Check sheet for the modelled part. Datum: model origin and axes. Units: mm. Round coordinates to 2 decimals unless told otherwise and drop trailing zeros.
Item 1: Material ranges on line 1 (Y direction, x = 0, z = 137); line 2 (X direction, y = -4.5, z = 201), recorded low to high.
Item 2: Release check for a two-part mould opening along X. For faces 1 (the cylindrical face through (-0.596, 2.685, 108.46)), 2 (the flat face through (6, 10, 108)), 3 (the flat face through (10, -6, 108)) record: +X half, -X half, draft (parallel to the pull), parting line (faces both ways), or undercut.
Item 3: Go/stop test with flat-tipped pins: pin 1 Ø3 at (x, y) = (2, -6) entering from +Z; pin 2 Ø1.5 at (y, z) = (0, 160.5) entering from +X; pin 3 Ø0.8 at (y, z) = (2, 73.5) entering from -X. Record where each tip stops, or that it passes through.
Autodesk Inventor part; units mm, degrees
ref_plane "Startebene" through (0, 0, 0) normal (0, 0, 1) x (1, 0, 0)
ref_plane "Endebene" through (0, 0, 320) normal (0, 0, 1) x (1, 0, 0)
ref_plane "Startebene1" through (0, 0, 0) normal (0, 0, 1) x (1, 0, 0)
ref_plane "Startebene" through (0, 0, 0) normal (0, 0, 1) x (1, 0, 0)
ref_plane "Endebene" through (0, 0, 320) normal (0, 0, 1) x (1, 0, 0)
ref_plane "Startebene1" through (0, 0, 0) normal (0, 0, 1) x (1, 0, 0)
ref_plane "Endebene1" through (0, 0, 220) normal (0, 0, 1) x (1, 0, 0)
ref_plane "Startebene2" through (0, 0, 0) normal (0, 0, 1) x (1, 0, 0)
ref_plane "Endebene2" through (0, 0, 220) normal (0, 0, 1) x (1, 0, 0)
sketch "Skizze" plane through (0, 0, 0) normal (0, 0, 1) x (1, 0, 0)
  line L0 (-10, 9) -> (-10, 3.3)
  arc A0 (-10, 3.3) -> (-9.7, 3) centre (-9.7, 3.3) ccw
  line L1 (-9.7, 3) -> (-8, 3)
  line L2 (-8, 3) -> (-8, 6)
  line L3 (-8, 6) -> (-7.0607, 6)
  line L4 (-7.0607, 6) -> (-4, 2.9393)
  line L5 (-4, 2.9393) -> (-4, 0.3)
  line L6 (-4, 0.3) -> (-3.7, 0)
  line L7 (-3.7, 0) -> (-4, -0.3)
  line L8 (-4, -0.3) -> (-4, -2.9393)
  line L9 (-4, -2.9393) -> (-7.0607, -6)
  line L10 (-7.0607, -6) -> (-8, -6)
  line L11 (-8, -6) -> (-8, -3)
  line L12 (-8, -3) -> (-9.7, -3)
  arc A1 (-9.7, -3) -> (-10, -3.3) centre (-9.7, -3.3) ccw
  line L13 (-10, -3.3) -> (-10, -9)
  arc A2 (-10, -9) -> (-9, -10) centre (-9, -9) ccw
  line L14 (-9, -10) -> (-3.3, -10)
  arc A3 (-3.3, -10) -> (-3, -9.7) centre (-3.3, -9.7) ccw
  line L15 (-3, -9.7) -> (-3, -8)
  line L16 (-3, -8) -> (-6, -8)
  line L17 (-6, -8) -> (-6, -7.0607)
  line L18 (-6, -7.0607) -> (-2.9393, -4)
  line L19 (-2.9393, -4) -> (-0.3, -4)
  line L20 (-0.3, -4) -> (0, -3.7)
  line L21 (0, -3.7) -> (0.3, -4)
  line L22 (0.3, -4) -> (2.9393, -4)
  line L23 (2.9393, -4) -> (6, -7.0607)
  line L24 (6, -7.0607) -> (6, -8)
  line L25 (6, -8) -> (3, -8)
  line L26 (3, -8) -> (3, -9.7)
  arc A4 (3, -9.7) -> (3.3, -10) centre (3.3, -9.7) ccw
  line L27 (3.3, -10) -> (9, -10)
  arc A5 (9, -10) -> (10, -9) centre (9, -9) ccw
  line L28 (10, -9) -> (10, -3.3)
  arc A6 (10, -3.3) -> (9.7, -3) centre (9.7, -3.3) ccw
  line L29 (9.7, -3) -> (8, -3)
  line L30 (8, -3) -> (8, -6)
  line L31 (8, -6) -> (7.0607, -6)
  line L32 (7.0607, -6) -> (4, -2.9393)
  line L33 (4, -2.9393) -> (4, -0.3)
  line L34 (4, -0.3) -> (3.7, 0)
  line L35 (3.7, 0) -> (4, 0.3)
  line L36 (4, 0.3) -> (4, 2.9393)
  line L37 (4, 2.9393) -> (7.0607, 6)
  line L38 (7.0607, 6) -> (8, 6)
  line L39 (8, 6) -> (8, 3)
  line L40 (8, 3) -> (9.7, 3)
  arc A7 (9.7, 3) -> (10, 3.3) centre (9.7, 3.3) ccw
  line L41 (10, 3.3) -> (10, 9)
  arc A8 (10, 9) -> (9, 10) centre (9, 9) ccw
  line L42 (9, 10) -> (3.3, 10)
  arc A9 (3.3, 10) -> (3, 9.7) centre (3.3, 9.7) ccw
  line L43 (3, 9.7) -> (3, 8)
  line L44 (3, 8) -> (6, 8)
  line L45 (6, 8) -> (6, 7.0607)
  line L46 (6, 7.0607) -> (2.9393, 4)
  line L47 (2.9393, 4) -> (0.3, 4)
  line L48 (0.3, 4) -> (0, 3.7)
  line L49 (0, 3.7) -> (-0.3, 4)
  line L50 (-0.3, 4) -> (-2.9393, 4)
  line L51 (-2.9393, 4) -> (-6, 7.0607)
  line L52 (-6, 7.0607) -> (-6, 8)
  line L53 (-6, 8) -> (-3, 8)
  line L54 (-3, 8) -> (-3, 9.7)
  arc A10 (-3, 9.7) -> (-3.3, 10) centre (-3.3, 9.7) ccw
  line L55 (-3.3, 10) -> (-9, 10)
  arc A11 (-9, 10) -> (-10, 9) centre (-9, 9) ccw
  circle A12 centre (0, 0) radius 2.75
  dimension "d2" = 5.5
  dimension "d3" = 10
  dimension "d4" = 10
  dimension "d5" = 5.7
  dimension "d6" = 5.7
  dimension "d7" = 1.7
  dimension "d8" = 3
  dimension "d9" = 0.3
  dimension "d10" = 90
  dimension "d11" = 45
  dimension "d12" = 45
  dimension "d13" = 45
  dimension "d14" = 90
  dimension "d15" = 90
  dimension "d16" = 45
  dimension "d17" = 45
  dimension "d18" = 45
  dimension "d19" = 45
  dimension "d20" = 90
  dimension "d21" = 90
  dimension "d22" = 45
  dimension "d23" = 45
  dimension "d24" = 90
  dimension "d25" = 90
  dimension "d26" = 90
  dimension "d27" = 90
  dimension "d28" = 90
  dimension "d29" = 90
  dimension "d30" = 90
  dimension "d31" = 90
  dimension "d32" = 90
  dimension "d33" = 90
  dimension "d34" = 90
  dimension "d35" = 90
  dimension "d36" = 90
  dimension "d37" = 90
  dimension "d38" = 90
  dimension "d39" = 4
  dimension "d40" = 6
  dimension "d41" = 13
  dimension "d42" = 14
  dimension "d43" = 16
  dimension "d44" = 18
  dimension "d45" = 3
  dimension "d46" = 9
  dimension "d47" = 7
  dimension "d48" = 1
  dimension "d49" = 7
  dimension "d50" = 1.5
  dimension "d51" = 1.8663
  dimension "d52" = 3.3663
  dimension "d53" = 1.5
  dimension "d54" = 1.8663
  dimension "d55" = 3.3663
  dimension "d56" = 4
  dimension "d57" = 10.8187
  dimension "d58" = 1.9092
  dimension "d59" = 5
  dimension "d60" = 13
  dimension "d61" = 13
  dimension "d62" = 16.0513
  dimension "d63" = 3.3234
  dimension "d64" = 14
  dimension "d65" = 12.685
extrude "Körper" add sketch "Skizze" along normal up to surface (220 mm away) from surface at 0
sketch "Skizze13" plane through (0, 0, 0) normal (0, 0, 1) x (1, 0, 0)
  line L0 (0, 0) -> (10, 0)
ref_plane "Arbeitsebene12" through (0, 0, 0) normal (0, -1, 0) x (1, 0, 0)
sketch "Skizze14" plane through (0, 0, 0) normal (0, -1, 0) x (1, 0, 0)
  line L0 (-2, 0) -> (12, 0)
  line L1 (-2, 220) -> (12, 220)
  dimension "d80" = 220
equation "\"G_OFFSET_START\" = 0"
equation "\"G_OFFSET_END\" = 0"
equation "\"G_L\" = d80"
equation "\"G_OFFSET_START1\" = 0"
equation "\"G_OFFSET_END1\" = 0"
equation "\"G_OFFSET_START2\" = 0"
equation "\"G_OFFSET_END2\" = 0"
properties part number "Alu Profil 20x20 - AP2020" material "Aluminium 6061"
Response values:
1. line 1: y = -3.7 to -2.75, 2.75 to 3.7
1. line 2: x = -10 to -8, -5.56 to -3.44, 3.44 to 5.56, 8 to 10
2. face 1: undercut
2. face 2: draft
2. face 3: +X half
3. pin 1: passes through
3. pin 2: stops at x = 4
3. pin 3: stops at x = -4
